Study the drawing (mm; zero at the part's minimum x, y, z) and answer. A direction names the side the tool comes from. Coordinates: 2 decimals unless noted, no trailing zeros. Order: outer loops, then holes, each group sorted by start corner. A loop starts at its lowest first (then second) coordinate and runs counter-clockwise, first axis right, second up. Notation, with made-up numbers: (15.25, 58.5) - (70.25, 58.5) arc R32 ccw to (70.25, 89.5) - close; hole circle Ø3 at (25, 5). An arc over 180 degrees is marked (long way). Write item = value, one per line.
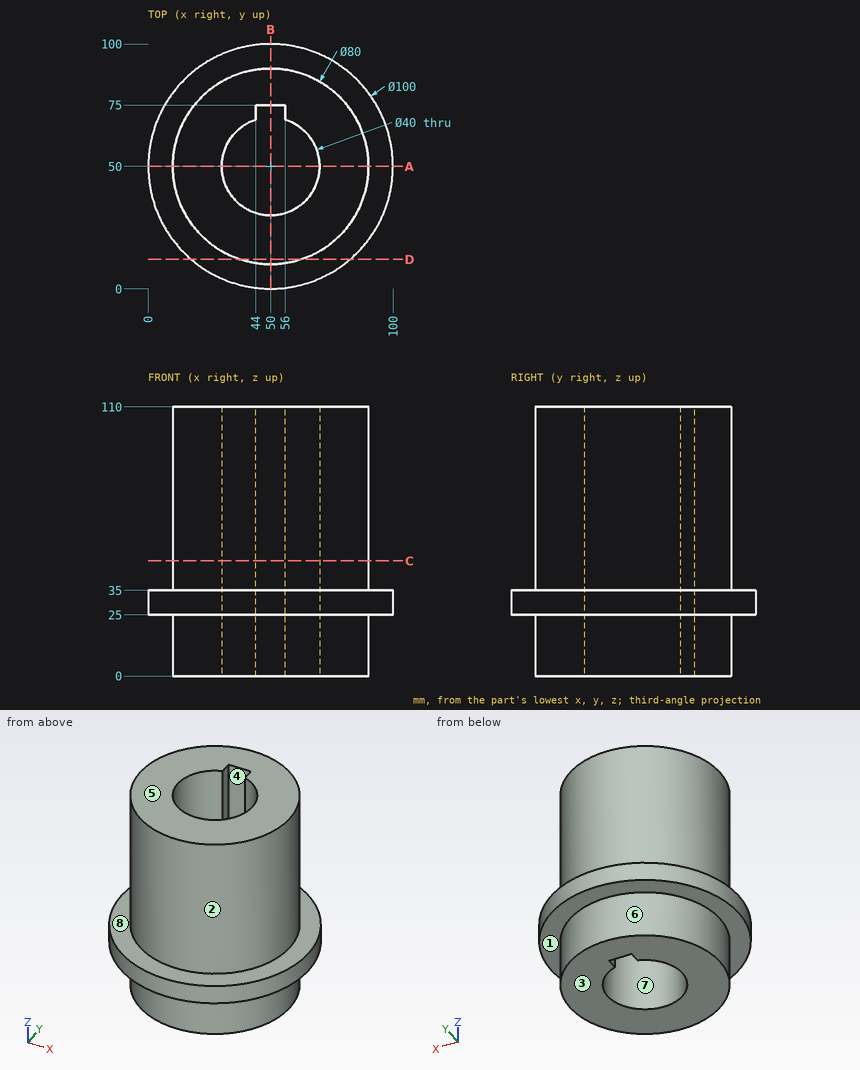
1) Flat-ended cylindrical pins translate along their axes: pin 1 Ø1 at (y, z) = (10, 31) entering from -X; pin 2 Ø3.5 at (x, z) = (47, 69.5) entering from -Y; pin 3 Ø3 at (x, y) = (72.5, 11.5) entering from -Z; pin 4 Ø24 at (x, y) = (50, 50) entering from +Z. Find the tip coordinate at first contact, or state that the pin passes through.
Returned:
pin_1 = 19.34
pin_2 = 10.02
pin_3 = 25
pin_4 = through
2) Straight lines are drawn through the part: line 1 along Y through (x, z) = (50, 79.5); line 2 along X through (y, z) = (50, 53); line 3 along Y through (x, z) = (50, 26.5). For each, find the intervals that lie inside material, in ascending order. Write a range as from..to.
Returned:
line_1 = 10..30, 75..90
line_2 = 10..30, 70..90
line_3 = 0..30, 75..100
3) The part is cut by section D-D (y = 12). Determine the outline of the cut face in (x, z), and give its area (3 significant figures).
Returned:
outline = (17.5, 25) - (37.51, 25) - (37.51, 0) - (62.49, 0) - (62.49, 25) - (82.5, 25) - (82.5, 35) - (62.49, 35) - (62.49, 110) - (37.51, 110) - (37.51, 35) - (17.5, 35) - close
area = 3,150 mm^2
4) The part is cut by section B-B (x = 50). Determine the outline of the cut face in (y, z), and give its area (3 significant figures).
Returned:
outline = (0, 25) - (10, 25) - (10, 0) - (30, 0) - (30, 110) - (10, 110) - (10, 35) - (0, 35) - close; (75, 0) - (90, 0) - (90, 25) - (100, 25) - (100, 35) - (90, 35) - (90, 110) - (75, 110) - close
area = 4,050 mm^2
5) Determine the mould class of the marked faces 6, 7 and 8 for opening direction X: pulls with the +X half, pulls with the -X half, needs draft (parallel to the pull), parting line crosses it, or undercut.
Returned:
face_6 = parting line crosses it
face_7 = undercut
face_8 = needs draft
6) The part is cut by section A-A (y = 50). Determine the outline of the cut face in (x, z), and give its area (3 significant figures).
Returned:
outline = (0, 25) - (10, 25) - (10, 0) - (30, 0) - (30, 110) - (10, 110) - (10, 35) - (0, 35) - close; (70, 0) - (90, 0) - (90, 25) - (100, 25) - (100, 35) - (90, 35) - (90, 110) - (70, 110) - close
area = 4,600 mm^2
7) The part is cut by section C-C (z = 47). Determine the outline of the cut face in (x, y).
Returned:
outline = circle Ø80 at (50, 50); hole (44, 69.08) arc R20 ccw (long way) to (56, 69.08) - (56, 75) - (44, 75) - close
8) For the marked faces 1, 2, 3, 4 and 5, determine the directions among +Z, -Z, +X, -X, +Y, -Y from which every point of the face is accessible in a straight line to the end or side of a thin tool.
Returned:
face_1 = -Z
face_2 = +Z
face_3 = -Z, +X, -X, +Y, -Y
face_4 = +Z, -Z
face_5 = +Z, +X, -X, +Y, -Y
